Could you check a few things on this model? Use its own coordinates, in mm. Face numbers are marked on the shaded views. A direction names the side the tool comes from. Round coordinates to 2 decimals unless told otherwise and drop trailing zeros. Write each loop counter-clockwise with the first axis right and the second up, starting at its lowest first coordinate (ties: lowest second). Pieces come first, ordered by that corner, then holes. Notation, with made-up numbers: (-28, 26.25) -> (-23, 26.25) arc R12 cw to (-23, 47.25) -> close; hole circle Ø4 at (3.5, 49.5). An arc over 180 degrees is marked (long way). Return JSON: item names as keys, results as strings.
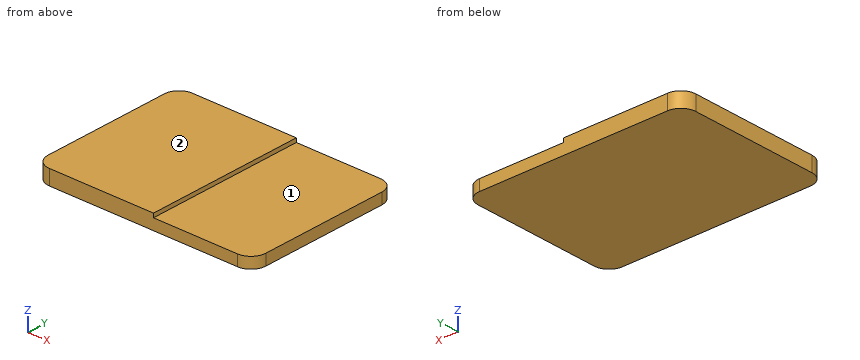
from build123d import *

# Parameters (mm, degrees)
F1_DEPTH = 80
F2_R     = 15


with BuildPart() as f1:
    # F0 (on Front) → F1 (new body, symmetric)
    with BuildSketch(Plane.XZ):
        Polygon((-110, -7.5), (110, -7.5), (110, 3.5), (10, 3.5), (10, 7.5), (-110, 7.5), align=None)
    extrude(amount=F1_DEPTH, both=True)

    # F2
    f2_edges = [f1.edges().sort_by_distance(p)[0] for p in [
        (-110, -80, 0),
        (110, -80, -2),
        (110, 80, -2),
        (-110, 80, 0),
    ]]
    fillet(f2_edges, radius=F2_R)


solid = f1.part
1) I want a section at A-A, the plane x = 35. Please give me the cut outline in (y, z), and give its area (3 significant figures).
Return value:
{"outline": "(-80, -7.5) -> (80, -7.5) -> (80, 3.5) -> (-80, 3.5) -> close", "area": "1,760 mm²"}
2) If I drill on probe 1 along Z at (x, y) = (81.5, 44); probe 2 along X at (y, z) = (-66, 0); probe 3 along X at (y, z) = (-21, 5.5), over which ranges is the centre line in solid material (lowest first)? Write a range as [from, to].
Return value:
{"probe 1": "[-7.5, 3.5]", "probe 2": "[-109.97, 109.97]", "probe 3": "[-110, 10]"}
3) I want a section at B-B, the plane y = 5.5. Please give me the cut outline in (x, z), and give its area (3 significant figures).
Return value:
{"outline": "(-110, -7.5) -> (110, -7.5) -> (110, 3.5) -> (10, 3.5) -> (10, 7.5) -> (-110, 7.5) -> close", "area": "2,900 mm²"}
4) Will these pins go through, and if not, where does the flat tip stop? pin 1 Ø12 at (x, y) = (54, -42) entering from +Z; pin 2 Ø1.2 at (y, z) = (21, 5.5) entering from +X.
Return value:
{"pin 1": "z = 3.5", "pin 2": "x = 10"}
5) For the marked faces 1 and 2, which set-ups out of +Z, -Z, +X, -X, +Y, -Y let a thin tool reach every point of the face, with its end or its side?
Return value:
{"face 1": "+Z, +X, +Y, -Y", "face 2": "+Z, +X, -X, +Y, -Y"}
